Work out the finished part from the listing and answer in its coordinate system (mm). A direction names the side the tool comes from. Round coordinates to 2 decimals unless told otherwise and drop trailing zeros. Order: outer loops, then holes, each group sorted by start corner. A loop starts at its lowest first (then second) coordinate and runs counter-clockwise, first axis right, second up.
from build123d import *

# Parameters (mm, degrees)
SKETCH1_W                   = 219.525
SKETCH1_H                   = 451
BOSS_EXTRUDE1_DEPTH         = 9.525
SKETCH2_W                   = 200.475
SKETCH2_H                   = 261.475
CUT_EXTRUDE1_DEPTH          = 6.525
FILLET1_R                   = 12.7
F_10_24_TAPPED_HOLE3_D      = 3.7973
F_10_24_TAPPED_HOLE1_D      = 3.7973
SKETCH9_R                   = 19.05
CUT_EXTRUDE2_DEPTH          = 4
F_6_CLEARANCE_HOLE1_D       = 3.6576
F_6_CLEARANCE_HOLE1_DEPTH   = 3
F_6_CLEARANCE_HOLE1_TIP     = 1.0988539
SKETCH12_R                  = 6.858
CUT_EXTRUDE3_DEPTH          = 4
F_10_CLEARANCE_HOLE1_D      = 4.9784
F_10_24_TAPPED_HOLE4_D      = 3.7973
F_10_24_TAPPED_HOLE4_DEPTH  = 18.03
F_10_24_TAPPED_HOLE4_TIP    = 1.140824014
F_10_CLEARANCE_HOLE2_D      = 5.1054
F_10_CLEARANCE_HOLE2_DEPTH  = 135.89
F_10_CLEARANCE_HOLE2_TIP    = 1.533816902
F_1_4_20_TAPPED_HOLE1_D     = 5.1054
F_1_4_20_TAPPED_HOLE1_DEPTH = 17.15
F_1_4_20_TAPPED_HOLE1_TIP   = 1.533816902


with BuildPart() as part:
    # Sketch1 → Boss-Extrude1 (new body)
    with BuildSketch(Plane(origin=(0, 0, 0), x_dir=(1, 0, 0), z_dir=(0, 1, 0))):
        Rectangle(SKETCH1_W, SKETCH1_H)
    extrude(amount=BOSS_EXTRUDE1_DEPTH)

    # Sketch2 → Cut-Extrude1 (cut)
    with BuildSketch(Plane(origin=(0, 9.525, 0), x_dir=(1, 0, 0), z_dir=(0, 1, 0))):
        with Locations((0, 85.2375)):
            Rectangle(SKETCH2_W, SKETCH2_H)
    extrude(amount=-CUT_EXTRUDE1_DEPTH, mode=Mode.SUBTRACT)

    # Fillet1
    fillet1_edges = [part.edges().sort_by_distance(p)[0] for p in [
        (-100.2375, 6.2625, -215.975),
        (100.2375, 6.2625, -215.975),
        (100.2375, 6.2625, 45.5),
        (-100.2375, 6.2625, 45.5),
    ]]
    fillet(fillet1_edges, radius=FILLET1_R)

    # #10-24 Tapped Hole3 (through all)
    with Locations(Plane(origin=(0, 9.525, 0), x_dir=(1, 0, 0), z_dir=(0, 1, 0))):
        with Locations((-8.7375, -59.5), (95.2625, -59.5), (-8.7375, -163.5), (95.2625, -163.5)):
            Hole(F_10_24_TAPPED_HOLE3_D / 2)

    # #10-24 Tapped Hole1 (through all)
    with Locations(Plane(origin=(0, 9.525, 0), x_dir=(1, 0, 0), z_dir=(0, 1, 0))):
        with Locations((83.2625, 220.7375), (3.2625, 220.7375)):
            Hole(F_10_24_TAPPED_HOLE1_D / 2)

    # Sketch9 → Cut-Extrude2 (cut, through all)
    with BuildSketch(Plane(origin=(0, 3, 0), x_dir=(1, 0, 0), z_dir=(0, 1, 0))):
        with Locations(Location((-62.1375, 177.875, 0), (0, 0, 270))):  # turned: the seam where the file's is
            Circle(SKETCH9_R)
    extrude(amount=-CUT_EXTRUDE2_DEPTH, mode=Mode.SUBTRACT)

    # #6 Clearance Hole1
    with Locations(Plane(origin=(0, 3, 0), x_dir=(1, 0, 0), z_dir=(0, 1, 0))):
        with Locations((-44.675, 195.3375), (-62.1375, 177.875), (-44.675, 160.4125), (-79.6, 160.4125), (-79.6, 195.3375)):
            Hole(F_6_CLEARANCE_HOLE1_D / 2, depth=F_6_CLEARANCE_HOLE1_DEPTH)
            with Locations((0, 0, -(F_6_CLEARANCE_HOLE1_DEPTH + F_6_CLEARANCE_HOLE1_TIP / 2))):  # 118° drill point
                Cone(0, F_6_CLEARANCE_HOLE1_D / 2, F_6_CLEARANCE_HOLE1_TIP, mode=Mode.SUBTRACT)

    # Sketch12 → Cut-Extrude3 (cut, through all)
    with BuildSketch(Plane(origin=(0, 3, 0), x_dir=(1, 0, 0), z_dir=(0, 1, 0))):
        with Locations(Location((-62.1375, 101.675, 0), (0, 0, 270))):  # turned: the seam where the file's is
            Circle(SKETCH12_R)
    extrude(amount=-CUT_EXTRUDE3_DEPTH, mode=Mode.SUBTRACT)

    # #10 Clearance Hole1 (through all)
    with Locations(Plane(origin=(0, 9.525, 0), x_dir=(1, 0, 0), z_dir=(0, 1, 0))):
        with Locations((105, 220.7375), (105, 0), (105, -220.7375)):
            Hole(F_10_CLEARANCE_HOLE1_D / 2)

    # #10-24 Tapped Hole4
    with Locations(Plane(origin=(0, 9.525, 0), x_dir=(1, 0, 0), z_dir=(0, 1, 0))):
        with Locations((-105, 206.45), (-105, 0), (-105, -206.45)):
            Hole(F_10_24_TAPPED_HOLE4_D / 2, depth=F_10_24_TAPPED_HOLE4_DEPTH)
            with Locations((0, 0, -(F_10_24_TAPPED_HOLE4_DEPTH + F_10_24_TAPPED_HOLE4_TIP / 2))):  # 118° drill point
                Cone(0, F_10_24_TAPPED_HOLE4_D / 2, F_10_24_TAPPED_HOLE4_TIP, mode=Mode.SUBTRACT)

    # #10 Clearance Hole2
    with Locations(Plane(origin=(0, 3, 0), x_dir=(1, 0, 0), z_dir=(0, 1, 0))):
        with Locations((-8.1625, 81.0375), (-8.1625, 33.4125), (48.9875, 123.9), (48.9875, -9.45)):
            Hole(F_10_CLEARANCE_HOLE2_D / 2, depth=F_10_CLEARANCE_HOLE2_DEPTH)
            with Locations((0, 0, -(F_10_CLEARANCE_HOLE2_DEPTH + F_10_CLEARANCE_HOLE2_TIP / 2))):  # 118° drill point
                Cone(0, F_10_CLEARANCE_HOLE2_D / 2, F_10_CLEARANCE_HOLE2_TIP, mode=Mode.SUBTRACT)

    # 1/4-20 Tapped Hole1
    with Locations(Plane(origin=(0, 9.525, 0), x_dir=(1, 0, 0), z_dir=(0, 1, 0))):
        with Locations((-16.7375, 220.7375)):
            Hole(F_1_4_20_TAPPED_HOLE1_D / 2, depth=F_1_4_20_TAPPED_HOLE1_DEPTH)
            with Locations((0, 0, -(F_1_4_20_TAPPED_HOLE1_DEPTH + F_1_4_20_TAPPED_HOLE1_TIP / 2))):  # 118° drill point
                Cone(0, F_1_4_20_TAPPED_HOLE1_D / 2, F_1_4_20_TAPPED_HOLE1_TIP, mode=Mode.SUBTRACT)


solid = part.part
Item 1: Find section B-B (y = 4.75). State how many separate pieces and enclosed holes the cut face has, plus the area to 3 significant figures.
Item 2: Find section A-A (x = 39.5). Write down the section's boundary in (y, z) (3 decimals).
Item 3: Find section C-C (z = -138). Write down the section's boundary in (x, y) (1 decimal).
Item 4: For a pull along Z with two mould halves and no side action, classify faces 3 (the face through (-2, 5, -225.5)), 4 (the face through (-2, 5, 225.5)), 5 (the face through (-109.762, 5, 3)), 6 (the face through (-96.42, 6.22, -212.35)) as released by +Z, released by -Z, zero draft, split by the parting line, or undercut.
Item 5: Find the intervals of material crossed by line 1 along X through (y, z) = (5.75, 59.5); line 2 along Z through (x, y) = (105, 7.75); line 3 along Z through (x, y) = (-105, 6), in increasing order.
Item 6: Given pin 1 (6 mm diameter, centred on x = -79.6, z = -160.41, fed in from +Y); pin 2 (3.5 mm diameter, centred on x = 95.26, z = 163.5, fed in from -Y), each flat-ended and moving along its own axis, determine where each tip first touches the part or whether it passes through.
Item 7: A tool of negligible diameter and unlimited length cuts with its end or side. For faces 1 (the face through (-64.76, 1.52, -95.34)), 2 (the face through (96.616, 6.217, -212.156)), from which of +Z, -Z, +X, -X, +Y, -Y can it reach the whole face along a straight path? Write none if from no direction.
Model answer:
1. separate pieces: 1
1. enclosed holes: 14
1. area: 46,500 mm2
2. outline: (0, -225.5) - (9.525, -225.5) - (9.525, -215.975) - (3, -215.975) - (3, 45.5) - (9.525, 45.5) - (9.525, 225.5) - (0, 225.5) - close
3. outline: (-109.8, 0) - (109.8, 0) - (109.8, 9.5) - (100.2, 9.5) - (100.2, 3) - (-100.2, 3) - (-100.2, 9.5) - (-109.8, 9.5) - close
4. face 3: released by -Z
4. face 4: released by +Z
4. face 5: zero draft
4. face 6: undercut
5. line 1: x = -109.76 to -10.64, -6.84 to 93.36, 97.16 to 109.76
5. line 2: z = -225.5 to -223.23, -218.25 to -2.49, 2.49 to 218.25, 223.23 to 225.5
5. line 3: z = -225.5 to -208.35, -204.55 to -1.9, 1.9 to 204.55, 208.35 to 225.5
6. pin 1: stops at y = 3
6. pin 2: passes through
7. face 1: +Y, -Y
7. face 2: +Y
